CAD build for the part. Positions are in the model's coordinates, mm. A direction names the side the tool comes from. Give positions to 0.01 mm unless a question says otherwise; leave off trailing zeros. Loops run counter-clockwise (first coordinate to the right, second up) from the corner with the lowest first, then second, coordinate; pieces in that order, holes last.
Item 1: Drop flat-ended pins along their axis: P1, Ø4, axis at x = 7.5, z = -6, coming from the +Y side; P2, Ø1.5, axis at y = -42.5, z = -7.5, coming from the -X side; P3, Ø4, axis at x = 9.5, z = -9, coming from the +Y side. Give the stop position or say it passes through.
Item 2: Mould opens along Y. For faces 3 (the cylindrical face through (0, 14, -8)), 4 (the conical face through (-2.472, -4.752, -3.516)), 5 (the cylindrical face through (-0.18, -36.39, -5.42)), 6 (the flat face through (14, -17, -8)) say: released by +Y, released by -Y, zero draft, split by the parting line, or undercut.
Item 3: Saw through at D-D on y = -22.5. Give the cut face in (x, z).
Item 4: Probe probe 1 along Y at (x, z) = (0, -8); probe 2 along Y at (x, z) = (0, -4.75); probe 3 along Y at (x, z) = (0, -5.5). List the from-to ranges inside material, lowest first.
Item 5: Saw through at C-C on z = -8.5. Give the cut face in (x, y), plus the area to 3 significant figures.
Item 6: Which spindle directions (+Z, -Z, +X, -X, +Y, -Y) get a long thin tool onto all of the face, cutting with end or side? Do faces 1 (the flat face through (-1, -39, -3.35)), 2 (the flat face through (2, 0, 0)). Say none if no direction does.
Item 7: Saw through at B-B on z = -1. Give the cut face in (x, y).
Item 8: Saw through at A-A on x = 0. Give the cut face in (y, z).
from build123d import *

# Parameters (mm, degrees)
SKETCH_1_R           = 3.9
SKETCH_1_R_2         = 1.4
EXTRUDE_1_DEPTH      = 3.35
SKETCH_2_R           = 5.2
SKETCH_3_R           = 7.7
EXTRUDE_2_DEPTH      = 5
MIRROR_START         = -3.35
MIRROR_6_OUTLINE_R   = 3.9
MIRROR_6_OUTLINE_R_2 = 1.4
MIRROR_6_DEPTH       = 3.35
SKETCH_1_3_R         = 1.4
CUT_EXTRUDE_1_DEPTH  = 11


# Read off the part's stored shape, not the designer's step: 镜向6
with BuildPart() as part:
    # 草图1 → 凸台-拉伸1 (new body)
    with BuildSketch(Plane.XY):
        Circle(SKETCH_1_R)
        Circle(SKETCH_1_R_2, mode=Mode.SUBTRACT)
    extrude(amount=-EXTRUDE_1_DEPTH)

    # 草图2 → 放样1 section 0
    with BuildSketch(Plane(origin=(0, 0, -3.35), x_dir=(-1, 0, 0), z_dir=(0, 0, -1))):
        Circle(SKETCH_2_R)
    # 草图3 → 放样1 section 1
    with BuildSketch(Plane(origin=(0, 0, -6), x_dir=(-1, 0, 0), z_dir=(0, 0, -1))):
        Circle(SKETCH_3_R)
    loft_1 = loft()

    # 草图5 → 凸台-拉伸2 (add)
    with BuildSketch(Plane(origin=(0, 0, -6), x_dir=(-1, 0, 0), z_dir=(0, 0, -1))):
        with BuildLine():
            Line((-14, 0), (-14, -35))
            ThreePointArc((-14, -35), (0, -49), (14, -35))
            Line((14, -35), (14, 0))
            ThreePointArc((14, 0), (0, 14), (-14, 0))
        make_face()
    extrude(amount=EXTRUDE_2_DEPTH)

    # 镜向5: 放样1 across plane
    add(loft_1.mirror(Plane(origin=(0, -17.5, 0), x_dir=(0, 0, 1), z_dir=(0, -1, 0))))

    # 镜向6 outline → 镜向6 (add)
    with BuildSketch(Plane.XY.offset(MIRROR_START)):
        with Locations((0, -35)):
            Circle(MIRROR_6_OUTLINE_R)
        with Locations((0, -35)):
            Circle(MIRROR_6_OUTLINE_R_2, mode=Mode.SUBTRACT)
    extrude(amount=MIRROR_6_DEPTH)

    # 草图1<3> → 切除-拉伸1 (cut)
    with BuildSketch(Plane.XY):
        Circle(SKETCH_1_3_R)
    cut_extrude_1 = extrude(amount=-CUT_EXTRUDE_1_DEPTH, mode=Mode.SUBTRACT)

    # 镜向7: 切除-拉伸1 across plane
    add(cut_extrude_1.mirror(Plane(origin=(0, -17.5, 0), x_dir=(0, 0, 1), z_dir=(0, -1, 0))), mode=Mode.SUBTRACT)


solid = part.part
Results below:
1. P1: stops at y = 12.87
1. P2: stops at x = -12.27
1. P3: stops at y = 11.82
2. face 3: released by +Y
2. face 4: undercut
2. face 5: undercut
2. face 6: zero draft
3. outline: (-14, -11) - (14, -11) - (14, -6) - (-14, -6) - close
4. probe 1: y = -49 to -36.4, -33.6 to -1.4, 1.4 to 14
4. probe 2: y = -41.52 to -36.4, -33.6 to -28.48, -6.52 to -1.4, 1.4 to 6.52
4. probe 3: y = -42.23 to -36.4, -33.6 to -27.77, -7.23 to -1.4, 1.4 to 7.23
5. outline: (-14, -35) arc R14 ccw to (14, -35) - (14, 0) arc R14 ccw to (-14, 0) - close; hole circle Ø2.8 at (0, -35); hole circle Ø2.8 at (0, 0)
5. area: 1,580 mm2
6. face 1: +Z
6. face 2: +Z, +X, -X, +Y, -Y
7. outline: circle Ø7.8 at (0, -35); circle Ø7.8 at (0, 0); hole circle Ø2.8 at (0, -35); hole circle Ø2.8 at (0, 0)
8. outline: (-49, -11) - (-36.4, -11) - (-36.4, 0) - (-38.9, 0) - (-38.9, -3.35) - (-40.2, -3.35) - (-42.7, -6) - (-49, -6) - close; (-33.6, -11) - (-1.4, -11) - (-1.4, 0) - (-3.9, 0) - (-3.9, -3.35) - (-5.2, -3.35) - (-7.7, -6) - (-27.3, -6) - (-29.8, -3.35) - (-31.1, -3.35) - (-31.1, 0) - (-33.6, 0) - close; (1.4, -11) - (14, -11) - (14, -6) - (7.7, -6) - (5.2, -3.35) - (3.9, -3.35) - (3.9, 0) - (1.4, 0) - close
